Here's how the part is built. I have some questions about the finished solid (model axes, mm). A direction names the side the tool comes from. Give positions to 0.01 mm unless a question says otherwise; leave off trailing zeros. Loops run counter-clockwise (first coordinate to the right, second up) from the corner with the lowest first, then second, coordinate; pieces in that order, holes last. Notation, with made-up numbers: (29, 26.25) - (86, 26.25) arc R21 cw to (86, 65.25) - close; hole circle Ø8 at (-34, -24). An arc over 180 degrees is marked (long way). Return JSON: item names as keys, results as strings. Group by question number.
(1) If we section it at C-C (z = -2.5): Please give me the cut outline in (x, y).
(2) I need wall thicknesses on probe 1 along X at (y, z) = (-1.5, -6.25); probe 2 along Z at (x, y) = (19, -4.75); probe 3 along Y at (x, z) = (21, -4.5). Which ranges of each line are inside material? Lowest first, please. Write a range as [from, to].
(3) If we section it at B-B (x = 8): Please give me the cut outline in (y, z).
(4) If we section it at D-D (x = -2.5): Please give me the cut outline in (y, z) (3 decimals), then the cut area to 3 significant figures.
(5) On a 3-axis mill with a long thin cutter (end or side, diameter ignored), from which of +Z, -Z, +X, -X, +Y, -Y can I reach the whole of each face in a straight line? I mean faces 1 (the flat face through (19.05, -6, -3)), 2 (the cylindrical face through (-3.22, 4.68, 4.29)), 3 (the flat face through (0, -6, 3)). Say none if no direction works.
(6) If we section it at A-A (y = -1): Please give me the cut outline in (x, z) (3 decimals), then the cut area to 3 significant figures.
(7) For P1, Ø6, axis at x = -1, z = -5, coming from the +Y side; P2, Ø3, axis at x = 18, y = -3, coming from the -Z side; P3, Ø4, axis at x = -1.5, y = -4.5, coming from the -Z side; P4, Ø1, axis at x = -1, z = 3, coming from the +Y side, each with a flat end and sliding along its axis, tell me the tip position at first contact or that it passes through.
```python
from build123d import *

# Parameters (mm, degrees)
BOSS_EXTRUDE1_DEPTH = 19.05
SKETCH2_R           = 6.35
BOSS_EXTRUDE2_DEPTH = 6.35
BOSS_EXTRUDE3_START = 6.35
SKETCH3_R           = 6.35
BOSS_EXTRUDE3_DEPTH = 6.35


with BuildPart() as part:
    # Sketch1 → Boss-Extrude1 (new body)
    with BuildSketch(Plane(origin=(0, 0, 0), x_dir=(0, 0, -1), z_dir=(1, 0, 0))):
        Polygon((-3.666174209, -6.35), (3.666174209, -6.35), (7.332348419, 0), (3.666174209, 6.35), (-3.666174209, 6.35), (-7.332348419, 0), align=None)
    extrude(amount=BOSS_EXTRUDE1_DEPTH)

    # Sketch2 → Boss-Extrude2 (add)
    with BuildSketch(Plane(origin=(19.05, 0, 0), x_dir=(0, 0, -1), z_dir=(1, 0, 0))):
        with Locations(Location((0, 0, 0), (0, 0, 150))):
            Circle(SKETCH2_R)
    extrude(amount=BOSS_EXTRUDE2_DEPTH)

    # Sketch3 → Boss-Extrude3 (add)
    with BuildSketch(Plane.ZY.offset(BOSS_EXTRUDE3_START)):
        with Locations(Location((0, 0, 0), (0, 0, 30))):
            Circle(SKETCH3_R)
    extrude(amount=-BOSS_EXTRUDE3_DEPTH)


solid = part.part
```
Values:
{
 "1": {"outline": "(-6.35, -5.84) - (0, -5.84) - (0, -6.35) - (19.05, -6.35) - (19.05, -5.84) - (25.4, -5.84) - (25.4, 5.84) - (19.05, 5.84) - (19.05, 6.35) - (0, 6.35) - (0, 5.84) - (-6.35, 5.84) - close"},
 "2": {"probe 1": "[0, 19.05]", "probe 2": "[-4.59, 4.59]", "probe 3": "[-4.48, 4.48]"},
 "3": {"outline": "(-6.35, -3.67) - (0, -7.33) - (6.35, -3.67) - (6.35, 3.67) - (0, 7.33) - (-6.35, 3.67) - close"},
 "4": {"outline": "circle Ø12.7 at (0, 0)", "area": "127 mm2"},
 "5": {"face 1": "-Z, +X, -Y", "face 2": "-X", "face 3": "+Z, -X, -Y"},
 "6": {"outline": "(-6.35, -6.271) - (0, -6.271) - (0, -6.755) - (19.05, -6.755) - (19.05, -6.271) - (25.4, -6.271) - (25.4, 6.271) - (19.05, 6.271) - (19.05, 6.755) - (0, 6.755) - (0, 6.271) - (-6.35, 6.271) - close", "area": "417 mm2"},
 "7": {"P1": "y = 6.35", "P2": "z = -6.47", "P3": "z = -5.84", "P4": "y = 5.84"}
}
